```python
from build123d import *

# Parameters (mm, degrees)
SKETCH1_R           = 12.7
SKETCH1_R_2         = 2.25
BOSS_EXTRUDE1_DEPTH = 3.175


with BuildPart() as part:
    # Sketch1 → Boss-Extrude1 (new body)
    with BuildSketch(Plane(origin=(0, 0, 0), x_dir=(1, 0, 0), z_dir=(0, 1, 0))):
        with BuildLine():
            ThreePointArc((-41.605402676, 12.224955819), (-47.252466269, -4.513280985), (-33, -14.95))
            ThreePointArc((-33, -14.95), (-20.2367226, -20.2367226), (-14.95, -33))
            ThreePointArc((-14.95, -33), (0, -47.95), (14.95, -33))
            ThreePointArc((14.95, -33), (20.2367226, -20.2367226), (33, -14.95))
            ThreePointArc((33, -14.95), (47.252466269, -4.513280985), (41.605402676, 12.224955819))
            ThreePointArc((41.605402676, 12.224955819), (0, 25.4), (-41.605402676, 12.224955819))
        make_face()
        Circle(SKETCH1_R, mode=Mode.SUBTRACT)
        with Locations((-33, 0)):
            Circle(SKETCH1_R_2, mode=Mode.SUBTRACT)
        with Locations((33, 0)):
            Circle(SKETCH1_R_2, mode=Mode.SUBTRACT)
        with Locations((0, -33)):
            Circle(SKETCH1_R_2, mode=Mode.SUBTRACT)
    extrude(amount=BOSS_EXTRUDE1_DEPTH)


solid = part.part
```
Check sheet for the modelled part. Datum: model origin and axes. Units: mm. Coordinates: 2 decimals unless noted, no trailing zeros. Loops run counter-clockwise (first coordinate to the right, second up) from the corner with the lowest first, then second, coordinate; pieces in that order, holes last. Notation, with made-up numbers: M 29,-23.5 L 45,-23.5 A26 ccw 45,4.5 Z; hole C -29.5,41.25 d2. An arc over 180 degrees is marked long. Answer as a JSON object with one key per item and string values.
1. Sectioned sample at D-D on z = 38. Record the cut outline in (x, y) (3 decimals), and give its area (3 significant figures).
Outcome:
{"outline": "M -14.089,0 L 14.089,0 L 14.089,3.175 L -14.089,3.175 Z", "area": "89.5 mm²"}
2. Sectioned sample at C-C on x = 0. Record the cut outline in (y, z) (3 decimals), and give its area (3 significant figures).
Outcome:
{"outline": "M 0,-25.4 L 3.175,-25.4 L 3.175,-12.7 L 0,-12.7 Z; M 0,12.7 L 3.175,12.7 L 3.175,30.75 L 0,30.75 Z; M 0,35.25 L 3.175,35.25 L 3.175,47.95 L 0,47.95 Z", "area": "138 mm²"}
3. Release check for a two-part mould opening along X. For faces 1 (the cylindrical face through (35.08, 1.57, 0.86)), 2 (the cylindrical face through (-20.378, 1.565, 20.097)), 3 (the cylindrical face through (47.17, 1.57, 4.76)), 4 (the flat face through (10, 3.175, 11)) record: pulls with the +X half, pulls with the -X half, needs draft (parallel to the pull), parting line crosses it, or undercut.
Outcome:
{"face 1": "undercut", "face 2": "pulls with the -X half", "face 3": "pulls with the +X half", "face 4": "needs draft"}
4. Sectioned sample at B-B on y = 1.9. Record the cut outline in (x, z), and give its area (3 significant figures).
Outcome:
{"outline": "M -41.61,-12.22 A72.28 ccw 41.61,-12.22 A14.95 ccw 33,14.95 A18.05 cw 14.95,33 A14.95 ccw -14.95,33 A18.05 cw -33,14.95 A14.95 ccw Z; hole C -33,0 d4.5; hole C 0,0 d25.4; hole C 0,33 d4.5; hole C 33,0 d4.5", "area": "3,690 mm²"}
5. Sectioned sample at A-A on z = 0. Record the cut outline in (x, y) (3 decimals).
Outcome:
{"outline": "M -47.95,0 L -35.25,0 L -35.25,3.175 L -47.95,3.175 Z; M -30.75,0 L -12.7,0 L -12.7,3.175 L -30.75,3.175 Z; M 12.7,0 L 30.75,0 L 30.75,3.175 L 12.7,3.175 Z; M 35.25,0 L 47.95,0 L 47.95,3.175 L 35.25,3.175 Z"}
6. Scan lines: L1, parallel to Z at x = 0, y = 1.35; L2, parallel to X at y = 1.8, z = 0; L3, parallel to Z at x = -1, y = 0.7. Record each from-to range of solid material in increasing order. Write a range as from..to.
Outcome:
{"L1": "-25.4..-12.7, 12.7..30.75, 35.25..47.95", "L2": "-47.95..-35.25, -30.75..-12.7, 12.7..30.75, 35.25..47.95", "L3": "-25.39..-12.66, 12.66..30.98, 35.02..47.92"}
7. Depth check by flat-ended pin: P1, Ø1, axis at y = 0.5, z = -11.5, coming from the +X side. Enter the tip coordinate at first touch or a pass-through.
Outcome:
{"P1": "x = 43.12"}
